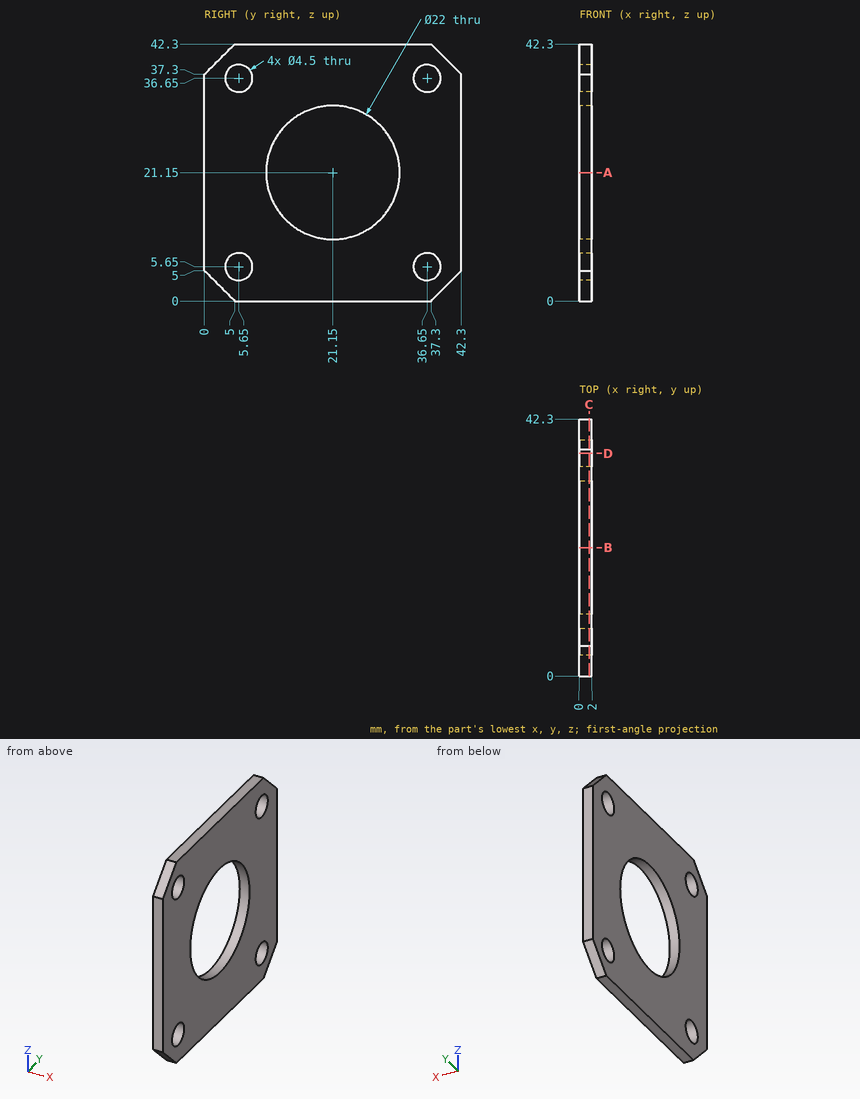
Here's the drawing with two shaded views (mm, measured from the low corner). I have some questions. Coordinates: 2 decimals unless noted, no trailing zeros. Write each loop counter-clockwise with the first axis right and the second up, starting at its lowest first coordinate (ties: lowest second). Pieces come first, ordered by that corner, then holes. Notation, with made-up numbers: M 85,69 L 140,69 A22 ccw 140,99 Z; hole C 63.25,-6 d5. An arc over 180 degrees is marked long. Write item = value, one per line. Start each with the question number.
Q1. If we section it at D-D, the plane y = 36.65: Write out the boundary of the cut face in (x, z).
Q2. If I drill on L1, parallel to Z at x = 1.35, y = 36.65; L2, parallel to Z at x = 0.65, y = 37.5; L3, parallel to Y at x = 0.1, z = 19, over which ranges is the centre line in solid material (lowest first)? Write a range as [from, to].
Q3. If we section it at C-C, the plane x = 1.6: Write out the boundary of the cut face in (y, z).
Q4. I'm going to push flat-ended pins straight in: pin 1 (2 mm diameter, centred on y = 7, z = 19.5, fed in from -X); pin 2 (3.5 mm diameter, centred on y = 36.65, z = 5.65, fed in from +X). Where does each tip first touch, or does it pass through?
Q5. If we section it at A-A, the plane z = 21.15: Write out the boundary of the cut face in (x, y), then the cut area to 3 significant figures.
Check sheet entries:
q1.outline = M 0,0 L 2,0 L 2,3.4 L 0,3.4 Z; M 0,7.9 L 2,7.9 L 2,34.4 L 0,34.4 Z; M 0,38.9 L 2,38.9 L 2,42.3 L 0,42.3 Z
q2.L1 = [0, 3.4], [7.9, 34.4], [38.9, 42.3]
q2.L2 = [0.2, 3.57], [7.73, 34.57], [38.73, 42.1]
q2.L3 = [0, 10.36], [31.94, 42.3]
q3.outline = M 0,5 L 5,0 L 37.3,0 L 42.3,5 L 42.3,37.3 L 37.3,42.3 L 5,42.3 L 0,37.3 Z; hole C 5.65,5.65 d4.5; hole C 5.65,36.65 d4.5; hole C 21.15,21.15 d22; hole C 36.65,5.65 d4.5; hole C 36.65,36.65 d4.5
q4.pin_1 = 0
q4.pin_2 = through
q5.outline = M 0,0 L 2,0 L 2,10.15 L 0,10.15 Z; M 0,32.15 L 2,32.15 L 2,42.3 L 0,42.3 Z
q5.area = 40.6 mm²
